Model file for the job. Use its own axes, mm. Face numbers are marked on the shaded views. A direction names the side the tool comes from. Coordinates: 2 decimals unless noted, no trailing zeros. Order: outer loops, then holes, each group sorted by start corner. A loop starts at its lowest first (then second) coordinate and runs counter-clockwise, first axis right, second up. Notation, with made-up numbers: (16, 41) -> (68, 41) arc R21 ccw to (68, 76) -> close; hole circle Ø7 at (53.25, 56.5). An arc over 180 degrees is marked (long way). Use CSV: the item, a comma, the result in double quotes. Start each with the question number.
(1) Probe L1, parallel to Y at x = -7, z = -21; L2, parallel to Z at x = 27.15, y = 15; L3, parallel to X at y = 19.5, z = -33.5. List the from-to ranges inside material, lowest first.
(2) Pull direction X, two halves, no side cores. Call the marked faces 4, 5 and 6: pulls with the +X half, pulls with the -X half, needs draft (parallel to the pull), parting line crosses it, or undercut.
(3) Cut at C-C on y = 15. Write the cut outline in (x, z).
(4) Cut at B-B on x = -7. Give the number of separate pieces and of enclosed holes in the cut face, plus the area to 3 significant figures.
(5) Cut at A-A on z = -10. Write the cut outline in (x, y), plus the area to 4 significant figures.
(6) Pin check, flat tips, straight feed: pin 1 Ø10 at (x, y) = (20, 25) entering from +Z; pin 2 Ø10 at (x, z) = (14.5, -11.5) entering from +Y; pin 3 Ø3 at (x, y) = (-4, 16) entering from -Z. Stop position of each tip, or through.
(7) Tool access for the marked faces 1, 2 and 3: list every direction of +Z, -Z, +X, -X, +Y, -Y with a clear straight run to the whole face (end or side of a thin tool).
(8) Cut at D-D on x = 27. Write the cut outline in (y, z), plus the area to 3 significant figures.
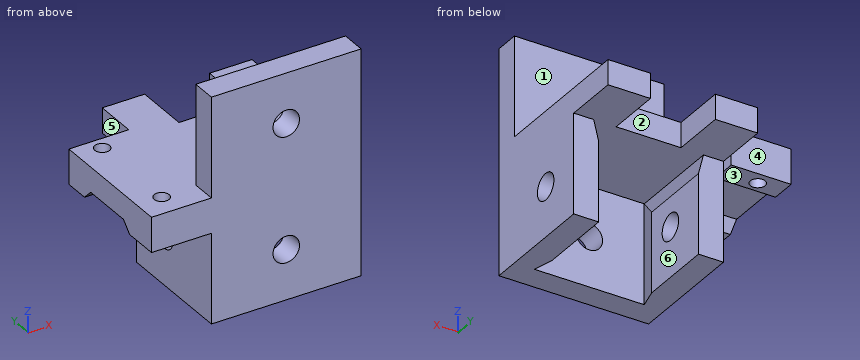
```python
from build123d import *

# Parameters (mm, degrees)
SKETCH1_W               = 30
SKETCH1_H               = 45
BOSS_EXTRUDE1_DEPTH     = 5
SKETCH2_W               = 30
SKETCH2_H               = 5
BOSS_EXTRUDE2_DEPTH     = 30
SKETCH3_W               = 5
SKETCH3_H               = 20
BOSS_EXTRUDE3_DEPTH     = 19
SKETCH4_W               = 13
SKETCH4_H               = 5
CUT_EXTRUDE1_DEPTH      = 11
SKETCH5_R               = 2.65
CUT_EXTRUDE2_DEPTH      = 10
CUT_EXTRUDE3_DEPTH      = 65.420493634
CUT_EXTRUDE3_DEPTH_BACK = 65.420493634
SKETCH6_R               = 2.65
CUT_EXTRUDE4_DEPTH      = 20
CUT_EXTRUDE5_REACH      = 61.169
SKETCH9_W               = 5
SKETCH9_H               = 26.5
BOSS_EXTRUDE4_DEPTH     = 12
SKETCH10_W              = 12
SKETCH10_H              = 9
SKETCH10_H_2            = 7
BOSS_EXTRUDE5_DEPTH     = 2
CHAMFER1_SIZE           = 2
CHAMFER2_SIZE           = 2
SKETCH11_R              = 1.5
CUT_EXTRUDE6_DEPTH      = 54.422841557


with BuildPart() as part:
    # Sketch1 → Boss-Extrude1 (new body)
    with BuildSketch(Plane(origin=(0, 0, 0), x_dir=(1, 0, 0), z_dir=(0, 1, 0))):
        with Locations((15, 22.5)):
            Rectangle(SKETCH1_W, SKETCH1_H)
    extrude(amount=BOSS_EXTRUDE1_DEPTH)

    # Sketch2 → Boss-Extrude2 (add)
    with BuildSketch(Plane(origin=(0, 5, 0), x_dir=(1, 0, 0), z_dir=(0, 1, 0))):
        with Locations((15, 22.5)):
            Rectangle(SKETCH2_W, SKETCH2_H)
    extrude(amount=BOSS_EXTRUDE2_DEPTH)

    # Sketch3 → Boss-Extrude3 (add)
    with BuildSketch(Plane(origin=(0, 5, 0), x_dir=(1, 0, 0), z_dir=(0, 1, 0))):
        with Locations((2.5, 35)):
            Rectangle(SKETCH3_W, SKETCH3_H)
        with Locations((27.5, 35)):
            Rectangle(SKETCH3_W, SKETCH3_H)
    extrude(amount=BOSS_EXTRUDE3_DEPTH)

    # Sketch4 → Cut-Extrude1 (cut)
    with BuildSketch(Plane(origin=(0, 35, 0), x_dir=(1, 0, 0), z_dir=(0, 1, 0))):
        with Locations((15, 22.5)):
            Rectangle(SKETCH4_W, SKETCH4_H)
    extrude(amount=-CUT_EXTRUDE1_DEPTH, mode=Mode.SUBTRACT)

    # Sketch5 → Cut-Extrude2 (cut)
    with BuildSketch(Plane.XZ):
        with Locations(Location((15, -10, 0), (0, 0, 270))):
            Circle(SKETCH5_R)
        with Locations(Location((15, -35, 0), (0, 0, 270))):
            Circle(SKETCH5_R)
    extrude(amount=-CUT_EXTRUDE2_DEPTH, mode=Mode.SUBTRACT)

    # Sketch6 → Cut-Extrude3 (cut, two sides: drawn at the far end of the back side and taken through both)
    with BuildSketch(Plane(origin=(30, 0, 0), x_dir=(0, 0, -1), z_dir=(1, 0, 0)).offset(-CUT_EXTRUDE3_DEPTH_BACK)):
        with Locations((35, 15)):
            Circle(SKETCH6_R)
    extrude(amount=CUT_EXTRUDE3_DEPTH + CUT_EXTRUDE3_DEPTH_BACK, mode=Mode.SUBTRACT)

    # Sketch7 → Cut-Extrude4 (cut)
    with BuildSketch(Plane(origin=(0, 0, -45), x_dir=(-1, 0, 0), z_dir=(0, 0, -1))):
        Polygon((-25, 5), (-26, 5), (-25, 9), align=None)
        Polygon((-5, 5), (-4, 5), (-5, 9), align=None)
    extrude(amount=-CUT_EXTRUDE4_DEPTH, mode=Mode.SUBTRACT)

    # Cut-Extrude5: up to this face of the body (flat: up to its plane)
    cut_extrude5_end = Plane(part.part.faces().sort_by_distance((0.360555128, 5, -10))[0])
    # Sketch8 → Cut-Extrude5 (cut, up to the picked face)
    with BuildSketch(Plane(origin=(0, 24, 0), x_dir=(1, 0, 0), z_dir=(0, 1, 0)), mode=Mode.PRIVATE) as cut_extrude5_sk1:
        Polygon((25, 25), (26, 25), (25, 29), align=None)
    cut_extrude5_tool1 = split(extrude(cut_extrude5_sk1.sketch, amount=-CUT_EXTRUDE5_REACH, mode=Mode.PRIVATE), bisect_by=cut_extrude5_end, keep=Keep.BOTH, mode=Mode.PRIVATE)
    # Sketch8 → Cut-Extrude5 (cut, up to the picked face)
    with BuildSketch(Plane(origin=(0, 24, 0), x_dir=(1, 0, 0), z_dir=(0, 1, 0)), mode=Mode.PRIVATE) as cut_extrude5_sk2:
        Polygon((5, 25), (5, 29), (4, 25), align=None)
    cut_extrude5_tool2 = split(extrude(cut_extrude5_sk2.sketch, amount=-CUT_EXTRUDE5_REACH, mode=Mode.PRIVATE), bisect_by=cut_extrude5_end, keep=Keep.BOTH, mode=Mode.PRIVATE)
    add(cut_extrude5_tool1.solids().sort_by(Axis((25.333333, 24, -26.333333), (0, -1, 0)))[0], mode=Mode.SUBTRACT)
    add(cut_extrude5_tool2.solids().sort_by(Axis((4.666667, 24, -26.333333), (0, -1, 0)))[0], mode=Mode.SUBTRACT)

    # Sketch9 → Boss-Extrude4 (add)
    with BuildSketch(Plane.ZY):
        with Locations((-22.5, 13.25)):
            Rectangle(SKETCH9_W, SKETCH9_H)
    extrude(amount=BOSS_EXTRUDE4_DEPTH)

    # Sketch10 → Boss-Extrude5 (add)
    with BuildSketch(Plane(origin=(0, 0, -25), x_dir=(-1, 0, 0), z_dir=(0, 0, -1))):
        with Locations((6, 4.5)):
            Rectangle(SKETCH10_W, SKETCH10_H)
        with Locations((6, 23)):
            Rectangle(SKETCH10_W, SKETCH10_H_2)
    extrude(amount=BOSS_EXTRUDE5_DEPTH)

    # Chamfer1
    chamfer1_edges = [part.edges().sort_by_distance(p)[0] for p in [
        (-6, 19.5, -27),
    ]]
    chamfer(chamfer1_edges, length=CHAMFER1_SIZE - 0.0001)  # a hair under: the kernel refuses the full size

    # Chamfer2
    chamfer2_edges = [part.edges().sort_by_distance(p)[0] for p in [
        (-6, 9, -27),
    ]]
    chamfer(chamfer2_edges, length=CHAMFER2_SIZE - 0.0001)  # a hair under: the kernel refuses the full size

    # Sketch11 → Cut-Extrude6 (cut, through all)
    with BuildSketch(Plane(origin=(0, 0, -27), x_dir=(-1, 0, 0), z_dir=(0, 0, -1))):
        with Locations((7, 23.8)):
            Circle(SKETCH11_R)
        with Locations((7, 4.75)):
            Circle(SKETCH11_R)
    extrude(amount=-CUT_EXTRUDE6_DEPTH, mode=Mode.SUBTRACT)


solid = part.part
```
Outcome:
1,L1,"0 to 3.25, 6.25 to 22.3, 25.3 to 26.5"
1,L2,"-45 to -37.65, -32.35 to -20"
1,L3,"0 to 5, 25 to 30"
2,face 4,"needs draft"
2,face 5,"pulls with the -X half"
2,face 6,"undercut"
3,outline,"(-12, -25) -> (0, -25) -> (0, -32.35) -> (5, -32.35) -> (5, -29) -> (4, -25) -> (26, -25) -> (25, -29) -> (25, -32.35) -> (30, -32.35) -> (30, -20) -> (-12, -20) -> close; (0, -45) -> (5, -45) -> (5, -37.65) -> (0, -37.65) -> close; (25, -45) -> (30, -45) -> (30, -37.65) -> (25, -37.65) -> close"
4,separate pieces,"3"
4,enclosed holes,"0"
4,area,"119 mm2"
5,outline,"(0, 0) -> (12.35, 0) -> (12.35, 5) -> (0, 5) -> close; (17.65, 0) -> (30, 0) -> (30, 5) -> (17.65, 5) -> close"
5,area,"123.5 mm2"
6,pin 1,"z = -20"
6,pin 2,"y = 5"
6,pin 3,"z = -25"
7,face 1,"+Z, +X, -X, +Y"
7,face 2,"+Z, -Z, +Y"
7,face 3,"-Z, -X, +Y, -Y"
8,outline,"(0, -45) -> (24, -45) -> (24, -25) -> (35, -25) -> (35, -20) -> (5, -20) -> (5, 0) -> (0, 0) -> close; hole circle Ø5.3 at (15, -35)"
8,area,"733 mm2"
